Design review of the part shown in the three views and the two pictorial views. Dimensions are in mm from the part's minimum x, y and z. A direction names the side the tool comes from. Coordinates: 2 decimals unless noted, no trailing zeros. Loops run counter-clockwise (first coordinate to the right, second up) from the corner with the lowest first, then second, coordinate; pieces in that order, holes last.
Q1. Add section C-C on y = 26. Give the boundary of the cut face in (x, z), and give its area (3 significant figures).
Q2. Draft analysis for pull direction Y (two halves, no side actions). For the marked faces 1, 2, 3 and 4, state which applies: released by +Y, released by -Y, zero draft, split by the parting line, or undercut.
Q3. Add section A-A on x = 8. Give the boundary of the cut face in (y, z), and give its area (3 significant figures).
Q4. For P1, Ø12, axis at y = 17, z = 5.5, coming from the -X side; P2, Ø5.5, axis at x = 48, z = 10, coming from the +Y side; P3, Ø3.5, axis at y = 34, z = 8, coming from the +X side; P4, Ø9, axis at x = 47, z = 8.5, coming from the +Y side, all flat-tipped, find the tip position at first contact; note any pin that passes through.
Q5. Machinability: for the marked faces 5, 6 and 7, which of the approach directions +Z, -Z, +X, -X, +Y, -Y give a long, thin tool a straight path to every point of the face, cutting with its end or side? Answer none if there is none.
Q6. Add section D-D on x = 25.5. Give the boundary of the cut face in (y, z).
Q7. Add section B-B on z = 10. Give the number of separate pieces and of enclosed holes in the cut face.
Q8. Wall thickness on probe 1 along X at (y, z) = (7.5, 10); probe 2 along Z at (x, y) = (48, 3); probe 3 along Y at (x, z) = (21.5, 10): over which ranges is each line inside the solid? List them lowest first.
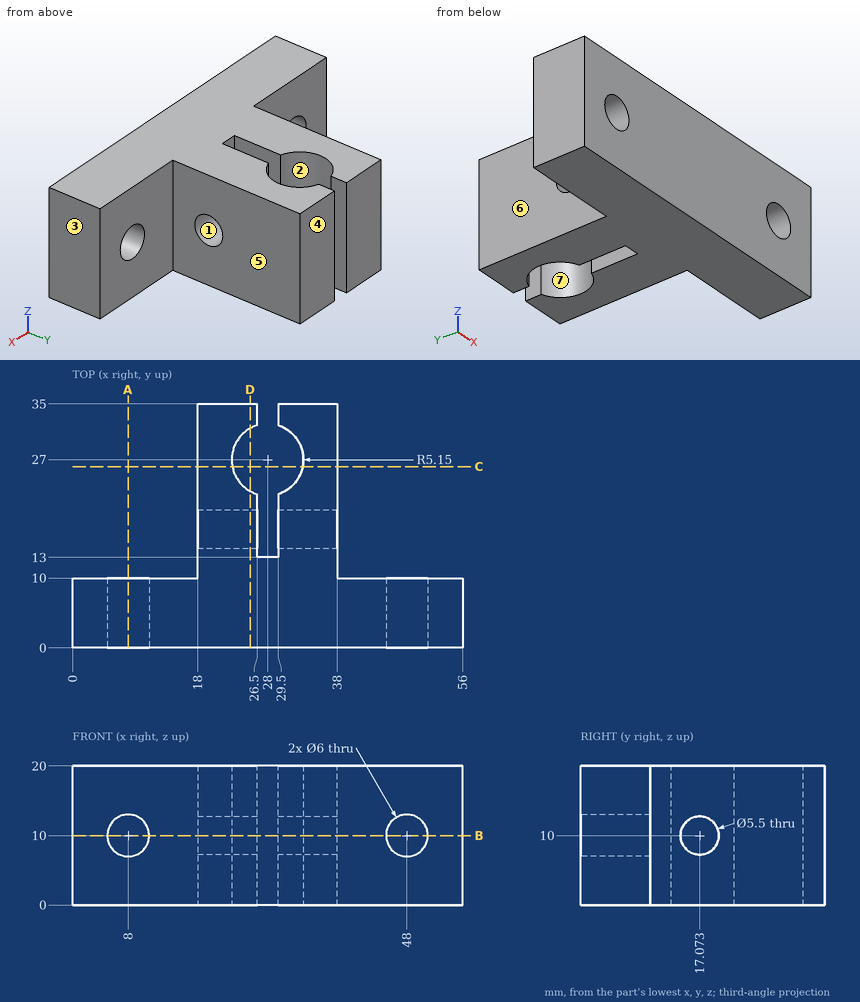
Entries:
1. outline: (18, 0) - (22.95, 0) - (22.95, 20) - (18, 20) - close; (33.05, 0) - (38, 0) - (38, 20) - (33.05, 20) - close
1. area: 198 mm2
2. face 1: undercut
2. face 2: undercut
2. face 3: zero draft
2. face 4: released by +Y
3. outline: (0, 0) - (10, 0) - (10, 7) - (0, 7) - close; (0, 13) - (10, 13) - (10, 20) - (0, 20) - close
3. area: 140 mm2
4. P1: stops at x = 18
4. P2: passes through
4. P3: stops at x = 38
4. P4: stops at y = 10
5. face 5: +Z, -Z, +X, +Y
5. face 6: +Z, -Z, -X, +Y
5. face 7: +Z, -Z
6. outline: (0, 0) - (22.5, 0) - (22.5, 20) - (0, 20) - close; (31.5, 0) - (35, 0) - (35, 20) - (31.5, 20) - close; hole circle Ø5.5 at (17.07, 10)
7. separate pieces: 5
7. enclosed holes: 0
8. probe 1: x = 0 to 5, 11 to 45, 51 to 56
8. probe 2: z = 0 to 7, 13 to 20
8. probe 3: y = 0 to 14.32, 19.82 to 35
